Drawing for the job (mm, zero at the part's lowest x, y, z). A direction names the side the tool comes from. Round coordinates to 2 decimals unless told otherwise and drop trailing zeros. Order: outer loops, then holes, each group sorted by start corner. A loop starts at its lowest first (then second) coordinate and runs counter-clockwise, first axis right, second up. Notation, with made-up numbers: M -40,-4.5 L 6,-4.5 A18 cw 6,21.5 Z; hole C -21,26.25 d6. An arc over 180 degrees is marked long. One line per item, written item: value. Start each with the question number.
Item 1: Tool access for the marked faces 1 and 2: list every direction of +Z, -Z, +X, -X, +Y, -Y with a clear straight run to the whole face (end or side of a thin tool).
Item 2: Pin check, flat tips, straight feed: pin 1 (4.5 mm diameter, centred on x = 121.54, z = 40, fed in from -Y); pin 2 (4 mm diameter, centred on x = 124.5, z = 105.5, fed in from -Y); pin 3 (6.5 mm diameter, centred on x = 69.85, z = 10.16, fed in from +Y); pin 4 (2 mm diameter, centred on x = 113.5, y = 9.5, fed in from +Z). Stop position of each tip, or through.
Item 3: Band-saw the part on A-A, the plane z = 10.16. Write the cut outline in (x, y).
Item 4: Band-saw the part on B-B, the plane x = 129.54. Write the cut outline in (y, z).
Item 5: Probe L1, parallel to Y at x = 34.5, z = 37.5 (1 decimal); L2, parallel to X at y = 15.5, z = 110 (1 decimal); L3, parallel to X at y = 8.25, z = 99 (1 decimal). List the from-to ranges inside material, lowest first.
Item 6: Band-saw the part on C-C, the plane z = 69.85. Give the number of separate pieces and of enclosed holes in the cut face, then the cut area to 3 significant figures.
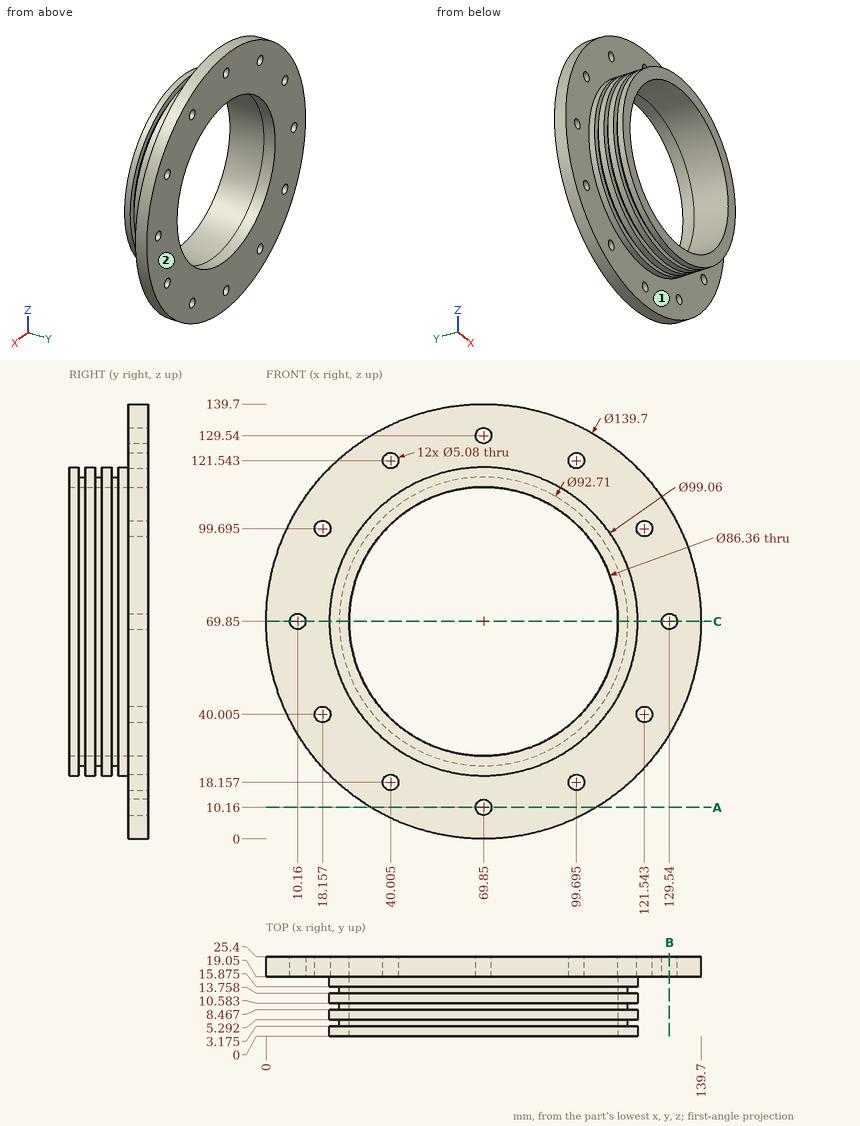
Output:
1. face 1: -Y
1. face 2: +Z, -Z, +X, -X, +Y
2. pin 1: passes through
2. pin 2: stops at y = 19.05
2. pin 3: stops at y = 25.4
2. pin 4: stops at z = 88.01
3. outline: M 33.57,19.05 L 67.31,19.05 L 67.31,25.4 L 33.57,25.4 Z; M 72.39,19.05 L 106.13,19.05 L 106.13,25.4 L 72.39,25.4 Z
4. outline: M 19.05,33.57 L 25.4,33.57 L 25.4,67.31 L 19.05,67.31 Z; M 19.05,72.39 L 25.4,72.39 L 25.4,106.13 L 19.05,106.13 Z
5. L1: y = 0 to 3.2, 5.3 to 8.5, 10.6 to 13.8, 15.9 to 25.4
5. L2: x = 46.7 to 54, 85.7 to 93
5. L3: x = 29.8 to 38, 101.7 to 109.9
6. separate pieces: 4
6. enclosed holes: 0
6. area: 476 mm²
